Here's how the part is built. I have some questions about the finished solid (model axes, mm). Face numbers are marked on the shaded views. A direction names the side the tool comes from. Round coordinates to 2 decimals unless told otherwise and drop trailing zeros. Order: outer loops, then holes, each group sorted by start corner. A loop starts at its lowest first (then second) coordinate and runs counter-clockwise, first axis right, second up. Notation, with made-up numbers: (55.25, -19) -> (77.25, -19) arc R25 ccw to (77.25, 9) -> close; hole circle Ø7 at (68, 29.25). An arc over 180 degrees is marked (long way). Use a Markdown table: item, result. Add a question column.
(1) I'm going to push flat-ended pins straight in: P1, Ø8, axis at x = 0, y = 8.5, coming from the +Z side; P2, Ø2, axis at y = 5, z = 2.5, coming from the -X side; P3, Ø1, axis at x = -2.5, y = 16, coming from the -Z side. Where does each tip first touch, or does it pass through?
(2) I want a section at D-D, the plane x = 3. Please give me the cut outline in (y, z), then the cut area to 3 significant figures.
(3) If I drill on probe 1 along Y at (x, z) = (0, 3.8); probe 2 along X at (y, z) = (7.62, -0.45); probe 3 along Y at (x, z) = (0, 0.5), over which ranges is the centre line in solid material (lowest first)?
(4) Thinking about a two-plate mould opening in Y: for the marked faces 1, 2 and 3, which applies, pulls with the +Y half, pulls with the -Y half, needs draft (parallel to the pull), parting line crosses it, or undercut?
(5) On a 3-axis mill with a long thin cutter (end or side, diameter ignored), from which of +Z, -Z, +X, -X, +Y, -Y can I reach the whole of each face in a straight line? I mean the marked faces 4 and 5. Say none if no direction works.
(6) I want a section at B-B, the plane y = 7.62. Please give me the cut outline in (x, z), then the cut area to 3 significant figures.
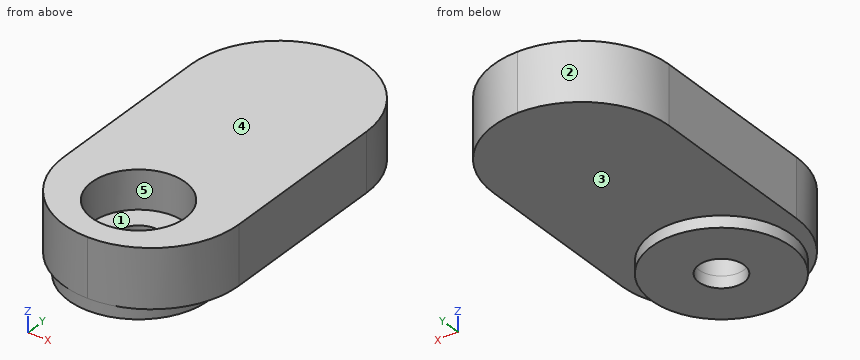
from build123d import *

# Parameters (mm, degrees)
SKETCH1_W                                      = 19.05
SKETCH1_H                                      = 38.1
BOSS_EXTRUDE1_DEPTH                            = 6.35
CBORE_FOR_8_SOCKET_HEAD_CAP_SCREW1_D           = 4.9149
CBORE_FOR_8_SOCKET_HEAD_CAP_SCREW1_CBORE_D     = 10.16
CBORE_FOR_8_SOCKET_HEAD_CAP_SCREW1_CBORE_DEPTH = 4.1656
BOSS_EXTRUDE2_START                            = 1.27
SKETCH4_R                                      = 7.62
SKETCH4_R_2                                    = 2.45745
BOSS_EXTRUDE2_DEPTH                            = 1.27
FILLET1_R                                      = 9.525


with BuildPart() as part:
    # Sketch1 → Boss-Extrude1 (new body)
    with BuildSketch(Plane.XY):
        with Locations((0, 19.05)):
            Rectangle(SKETCH1_W, SKETCH1_H)
    extrude(amount=BOSS_EXTRUDE1_DEPTH)

    # CBORE for #8 Socket Head Cap Screw1 (through all)
    with Locations(Plane.XY.offset(6.35)):
        with Locations((0, 7.62)):
            CounterBoreHole(CBORE_FOR_8_SOCKET_HEAD_CAP_SCREW1_D / 2, CBORE_FOR_8_SOCKET_HEAD_CAP_SCREW1_CBORE_D / 2, CBORE_FOR_8_SOCKET_HEAD_CAP_SCREW1_CBORE_DEPTH)

    # Sketch4 → Boss-Extrude2 (add)
    with BuildSketch(Plane(origin=(0, 0, 0), x_dir=(-1, 0, 0), z_dir=(0, 0, -1)).offset(BOSS_EXTRUDE2_START)):
        with Locations(Location((0, 7.62, 0), (0, 0, 270))):
            Circle(SKETCH4_R)
        with Locations(Location((0, 7.62, 0), (0, 0, 180))):
            Circle(SKETCH4_R_2, mode=Mode.SUBTRACT)
    extrude(amount=-BOSS_EXTRUDE2_DEPTH)

    # Fillet1
    fillet1_edges = [part.edges().sort_by_distance(p)[0] for p in [
        (9.525, 38.1, 3.175),
        (-9.525, 38.1, 3.175),
        (9.525, 0, 3.175),
        (-9.525, 0, 3.175),
    ]]
    fillet(fillet1_edges, radius=FILLET1_R - 0.0001)  # a hair under: the kernel refuses the full size


solid = part.part
Taken from the geometry:
| question | item | result |
|---|---|---|
| 1 | P1 | stops at z = 2.18 |
| 1 | P2 | stops at x = -8.85 |
| 1 | P3 | stops at z = 0 |
| 2 | outline | (0.48, 0) -> (0.62, 0) -> (0.62, -1.27) -> (14.62, -1.27) -> (14.62, 0) -> (37.62, 0) -> (37.62, 6.35) -> (11.72, 6.35) -> (11.72, 2.18) -> (3.52, 2.18) -> (3.52, 6.35) -> (0.48, 6.35) -> close |
| 2 | area | 219 mm2 |
| 3 | probe 1 | y = 0 to 2.54, 12.7 to 38.1 |
| 3 | probe 2 | x = -7.62 to -2.46, 2.46 to 7.62 |
| 3 | probe 3 | y = 0 to 5.16, 10.08 to 38.1 |
| 4 | face 1 | undercut |
| 4 | face 2 | pulls with the +Y half |
| 4 | face 3 | needs draft |
| 5 | face 4 | +Z, +X, -X, +Y, -Y |
| 5 | face 5 | +Z |
| 6 | outline | (-9.33, 0) -> (-7.62, 0) -> (-7.62, -1.27) -> (-2.46, -1.27) -> (-2.46, 2.18) -> (-5.08, 2.18) -> (-5.08, 6.35) -> (-9.33, 6.35) -> close; (2.46, -1.27) -> (7.62, -1.27) -> (7.62, 0) -> (9.33, 0) -> (9.33, 6.35) -> (5.08, 6.35) -> (5.08, 2.18) -> (2.46, 2.18) -> close |
| 6 | area | 78.6 mm2 |
